```python
from build123d import *

# Parameters (mm, degrees)
F0_W     = 1092.2
F0_H     = 838.2
F1_DEPTH = 19.05
F2_W     = 1054.1
F2_H     = 254
F3_DEPTH = 387.35
F5_DEPTH = 19.05


with BuildPart() as f1:
    # F0 (on Front) → F1 (new body)
    with BuildSketch(Plane.XZ):
        with Locations((8.787813, 419.1)):
            Rectangle(F0_W, F0_H)
    extrude(amount=F1_DEPTH)

    # F2 (on face) → F3 (join)
    with BuildSketch(Plane(origin=(0, 0, 0), x_dir=(-1, 0, 0), z_dir=(0, 1, 0))):
        Polygon((537.312187, 0), (537.312187, 838.2), (518.262187, 838.2), (-535.837813, 838.2), (-554.887813, 838.2), (-554.887813, 0), (-535.837813, 0), (-535.837813, 273.05), (518.262187, 273.05), (518.262187, 0), align=None)
        with Locations((-8.787813, 419.1)):
            Rectangle(F2_W, F2_H, mode=Mode.SUBTRACT)
        with Locations((-8.787813, 692.15)):
            Rectangle(F2_W, F2_H, mode=Mode.SUBTRACT)
    extrude(amount=F3_DEPTH)

    # F4 (on face) → F5 (cut)
    with BuildSketch(Plane.XY.offset(292.1)):
        with BuildLine():
            Line((-435.712187, 25.4), (-435.712187, 0))
            Line((-435.712187, 0), (-308.712187, 0))
            Line((-308.712187, 0), (-308.712187, 25.4))
            ThreePointArc((-308.712187, 25.4), (-312.431931, 34.380256), (-321.412187, 38.1))
            Line((-321.412187, 38.1), (-423.012187, 38.1))
            ThreePointArc((-423.012187, 38.1), (-431.992444, 34.380256), (-435.712187, 25.4))
        make_face()
        with BuildLine():
            Line((-54.712187, 25.4), (-54.712187, 0))
            Line((-54.712187, 0), (72.287813, 0))
            Line((72.287813, 0), (72.287813, 25.4))
            ThreePointArc((72.287813, 25.4), (68.568069, 34.380256), (59.587813, 38.1))
            Line((59.587813, 38.1), (-42.012187, 38.1))
            ThreePointArc((-42.012187, 38.1), (-50.992444, 34.380256), (-54.712187, 25.4))
        make_face()
        with BuildLine():
            Line((326.287813, 25.4), (326.287813, 0))
            Line((326.287813, 0), (453.287813, 0))
            Line((453.287813, 0), (453.287813, 25.4))
            ThreePointArc((453.287813, 25.4), (449.568069, 34.380256), (440.587813, 38.1))
            Line((440.587813, 38.1), (338.987813, 38.1))
            ThreePointArc((338.987813, 38.1), (330.007556, 34.380256), (326.287813, 25.4))
        make_face()
    extrude(amount=-F5_DEPTH, mode=Mode.SUBTRACT)


solid = f1.part
```
Could you check a few things on this model? Use its own coordinates, in mm. A direction names the side the tool comes from. Coordinates: 2 decimals unless noted, no trailing zeros. Write each loop counter-clockwise with the first axis right and the second up, starting at its lowest first coordinate (ties: lowest second). Pieces come first, ordered by that corner, then holes. Notation, with made-up numbers: (37.25, 22) -> (74.25, 22) arc R9 ccw to (74.25, 39) -> close; hole circle Ø3 at (28, -33.75). An arc over 180 degrees is marked (long way). One line per question, with ' | ' between items. Start each with the question number.
1. For faces 4 (the face through (254, -12, 0)), 5 (the face through (16, 191, 273.05)), 6 (the face through (535.838, 191, 417)), which set-ups out of +Z, -Z, +X, -X, +Y, -Y let a thin tool reach every point of the face, with its end or its side?
2. Thinking about a two-plate mould opening in X: for faces 1 (the face through (-537.312, 181, 413)), 2 (the face through (1, -19.05, 425)), 3 (the face through (16, 191, 546.1)), which applies, pulls with the +X half, pulls with the -X half, needs draft (parallel to the pull), parting line crosses it, or undercut?
3. If we section it at B-B (y = 106): Please give me the cut outline in (x, z), and give its area (3 significant figures).
4. If we section it at A-A (x = 14.5): Please give me the cut outline in (y, z), and give its area (3 significant figures).
5. If we section it at D-D (z = 233.5): Please give me the cut outline in (x, y), and give its area (3 significant figures).
6. Please list where these lines run through material, in increasing order: line 1 along Z through (x, y) = (72, 243.5); line 2 along X through (y, z) = (3, 254); line 3 along X through (y, z) = (27, 276).
7. Will these pins go through, and if not, where does the flat tip stop? P1, Ø10, axis at x = 200, z = 608.5, coming from the +Y side; P2, Ø1, axis at x = 69.5, y = 153.5, coming from the -Z side.
8. If we section it at C-C (x = -283): Please give me the cut outline in (y, z), and give its area (3 significant figures).
Return value:
1) face 4: -Z, +X, -X, +Y, -Y | face 5: -Z, +Y | face 6: +Y
2) face 1: pulls with the -X half | face 2: needs draft | face 3: undercut
3) outline: (-537.31, 0) -> (-518.26, 0) -> (-518.26, 273.05) -> (535.84, 273.05) -> (535.84, 0) -> (554.89, 0) -> (554.89, 838.2) -> (-537.31, 838.2) -> close; hole (-518.26, 292.1) -> (535.84, 292.1) -> (535.84, 546.1) -> (-518.26, 546.1) -> close; hole (-518.26, 565.15) -> (535.84, 565.15) -> (535.84, 819.15) -> (-518.26, 819.15) -> close | area: 92,200 mm²
4) outline: (-19.05, 0) -> (0, 0) -> (0, 546.1) -> (387.35, 546.1) -> (387.35, 565.15) -> (0, 565.15) -> (0, 819.15) -> (387.35, 819.15) -> (387.35, 838.2) -> (-19.05, 838.2) -> close; (38.1, 273.05) -> (387.35, 273.05) -> (387.35, 292.1) -> (38.1, 292.1) -> close | area: 37,400 mm²
5) outline: (-537.31, -19.05) -> (554.89, -19.05) -> (554.89, 387.35) -> (535.84, 387.35) -> (535.84, 0) -> (-518.26, 0) -> (-518.26, 387.35) -> (-537.31, 387.35) -> close | area: 35,600 mm²
6) line 1: z = 273.05 to 292.1, 546.1 to 565.15, 819.15 to 838.2 | line 2: x = -537.31 to -518.26, 535.84 to 554.89 | line 3: x = -537.31 to -435.61, -308.81 to -54.61, 72.19 to 326.39, 453.19 to 554.89
7) P1: stops at y = 0 | P2: stops at z = 273.05
8) outline: (-19.05, 0) -> (0, 0) -> (0, 273.05) -> (387.35, 273.05) -> (387.35, 292.1) -> (0, 292.1) -> (0, 546.1) -> (387.35, 546.1) -> (387.35, 565.15) -> (0, 565.15) -> (0, 819.15) -> (387.35, 819.15) -> (387.35, 838.2) -> (-19.05, 838.2) -> close | area: 38,100 mm²
